The model under review builds one solid part; all positions refer to its coordinate system, in mm. A direction names the side the tool comes from. Coordinates: 2 decimals unless noted, no trailing zeros. Loops run counter-clockwise (first coordinate to the right, second up) from the corner with the lowest first, then second, coordinate; pieces in that order, holes last. Notation, with made-up numbers: M 85.25,32 L 132.25,32 A26 ccw 132.25,64 Z; hole C 36,79.5 d8. An arc over 180 degrees is marked long. Write item = value, one per line. Start each with the question number.
Q1. We need section B-B on x = 0. Give the boundary of the cut face in (y, z) (1 decimal), and give its area (3 significant figures).
Q2. We need section D-D on z = -1. Give the boundary of the cut face in (x, y), and give its area (3 significant figures).
Q3. Wall thickness on probe 1 along Y at (x, z) = (0, 10); probe 2 along Y at (x, z) = (0, 1.75); probe 3 along Z at (x, y) = (4.9, 0): over which ranges is each line inside the solid? List them lowest first.
Q4. Clearance check with flat-ended pins moving along their axes: pin 1 Ø10 at (y, z) = (5.5, 12) entering from +X; pin 2 Ø8 at (x, z) = (1.5, 8) entering from -Y; pin 3 Ø1.5 at (x, z) = (-3, 2.5) entering from +Y. State where each tip first meets the part, or that it passes through.
Q5. We need section A-A on y = 0. Give the boundary of the cut face in (x, z) (1 decimal).
Q6. For faces 1 (the face through (-2.07, -9.31, 1.98)), 2 (the face through (5.53, 0.34, 9.54)), list the 3-axis set-ups (+Z, -Z, +X, -X, +Y, -Y) from which the entire face can be reached by the end or side of a thin tool; tool diameter is ignored.
Q7. Mouldability with a two-part tool opening along Y and no side actions: class faces 3 (the face through (-1.72, -7.75, 8.64)), 4 (the face through (2, 8, 2.381)), 5 (the face through (-0.414, 3.154, 6.472)) as released by +Y, released by -Y, zero draft, split by the parting line, or undercut.
Q8. We need section C-C on z = 6. Give the boundary of the cut face in (x, y) (1 decimal), and give its area (3 significant figures).
from build123d import *

# Parameters (mm, degrees)
SKETCH2_R           = 7.9375
BOSS_EXTRUDE1_DEPTH = 12.7
HOLE1_D             = 6.3627
SKETCH5_W           = 0.8763
SKETCH5_H           = 6.479418435


with BuildPart() as part:
    # Sketch1 → Revolve1 (revolve)
    with BuildSketch(Plane(origin=(0, 0, 0), x_dir=(1, 0, 0), z_dir=(0, 1, 0))):
        with BuildLine():
            Line((9.5377, 2.38125), (0, 2.38125))
            Line((0, 2.38125), (0, -2.38125))
            Line((0, -2.38125), (9.5377, -2.38125))
            Line((9.5377, -2.38125), (9.5377, -1.5875))
            ThreePointArc((9.5377, -1.5875), (7.9502, 0), (9.5377, 1.5875))
            Line((9.5377, 1.5875), (9.5377, 2.38125))
        make_face()
    revolve(axis=Axis((0, 0, -2.38125), (0, 0, 1)))

    # Sketch2 → Boss-Extrude1 (add)
    with BuildSketch(Plane.XY.offset(2.38125)):
        Circle(SKETCH2_R)
    extrude(amount=BOSS_EXTRUDE1_DEPTH)

    # Hole1 (through all)
    with Locations(Plane(origin=(0, 0, -2.38125), x_dir=(-1, 0, 0), z_dir=(0, 0, -1))):
        with Locations((0, 0)):
            Hole(HOLE1_D / 2)

    # Sketch5 → M1.6 Clearance Hole1 (revolve, cut)
    with BuildSketch(Plane(origin=(3.058281565, 0, 8.73125), x_dir=(0, 0, 1), z_dir=(0, 1, 0))):
        with Locations((0.43815, 3.239709218)):
            Rectangle(SKETCH5_W, SKETCH5_H)
    revolve(axis=Axis((-3.291718435, 0, 8.73125), (1, 0, 0)), mode=Mode.SUBTRACT)


solid = part.part
Returned:
q1.outline = M -9.5,-2.4 L -3.2,-2.4 L -3.2,15.1 L -7.9,15.1 L -7.9,2.4 L -9.5,2.4 L -9.5,1.6 A1.6 cw -9.5,-1.6 Z; M 3.2,-2.4 L 9.5,-2.4 L 9.5,-1.6 A1.6 cw 9.5,1.6 L 9.5,2.4 L 7.9,2.4 L 7.9,15.1 L 3.2,15.1 Z
q1.area = 173 mm^2
q2.outline = C 0,0 d16.61; hole C 0,0 d6.36
q2.area = 185 mm^2
q3.probe_1 = -7.94 to -3.18, 3.18 to 7.94
q3.probe_2 = -9.54 to -3.18, 3.18 to 9.54
q3.probe_3 = -2.38 to 7.85, 9.61 to 15.08
q4.pin_1 = 7.92
q4.pin_2 = -7.94
q4.pin_3 = 9.27
q5.outline = M -9.5,-2.4 L -3.2,-2.4 L -3.2,15.1 L -7.9,15.1 L -7.9,2.4 L -9.5,2.4 L -9.5,1.6 A1.6 cw -9.5,-1.6 Z; M 3.2,-2.4 L 9.5,-2.4 L 9.5,-1.6 A1.6 cw 9.5,1.6 L 9.5,2.4 L 7.9,2.4 L 7.9,7.9 L 3.2,7.9 Z; M 3.2,9.6 L 7.9,9.6 L 7.9,15.1 L 3.2,15.1 Z
q6.face_1 = +Z, -Z
q6.face_2 = +X
q7.face_3 = split by the parting line
q7.face_4 = zero draft
q7.face_5 = undercut
q8.outline = C 0,0 d15.9; hole C 0,0 d6.4
q8.area = 166 mm^2
